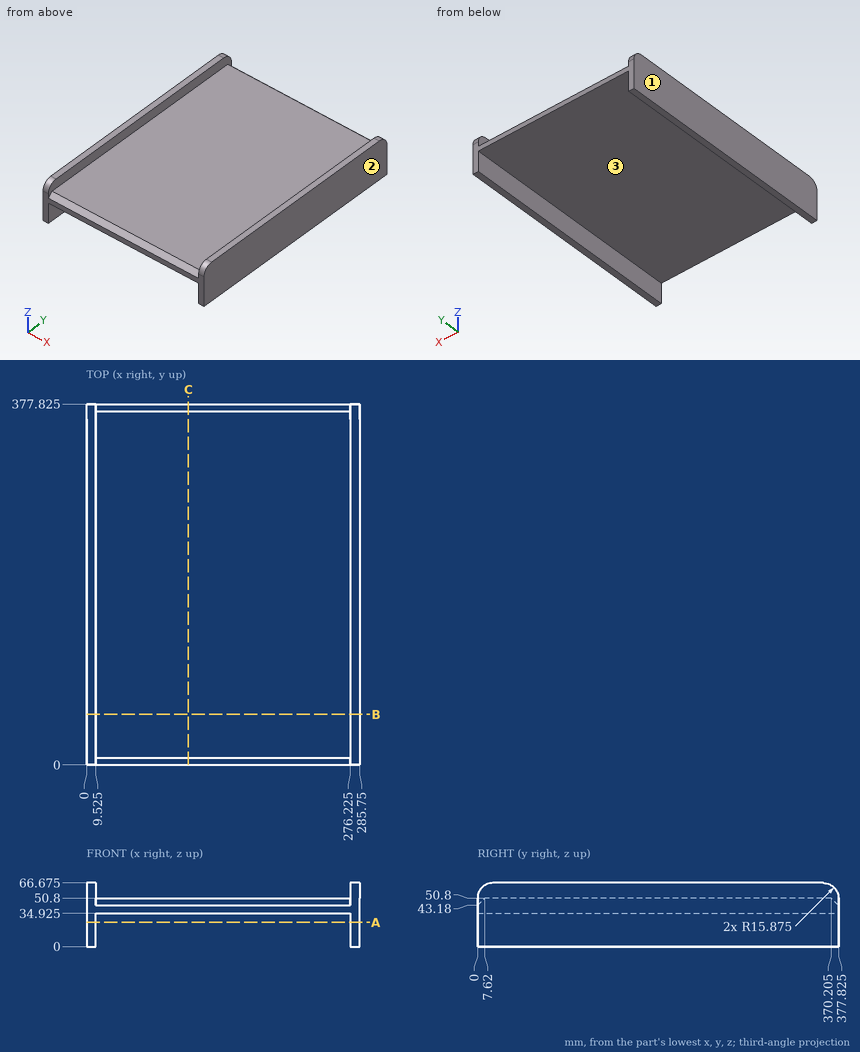
Geometry: see drawing. Coordinates: mm, zero at the bounding-box minimum. Give positions to 0.01 mm unless a question says otherwise; leave off trailing zeros. Write each loop counter-clockwise with the first axis right and the second up, starting at its lowest first coordinate (ties: lowest second). Pieces come first, ordered by that corner, then holes. Notation, with made-up numbers: M 62,-33 L 121,-33 A20 cw 121,-22 Z; hole C 53.5,58.25 d3. An arc over 180 degrees is marked long. Answer in a Markdown table with one row per item. Add a question column.
(1) Section C-C on x = 106.5. Return loops of the section in (y, z) (3 decimals), and give its area (3 significant figures).
(2) Section B-B on y = 53. Return loops of the section in (x, z) (3 decimals).
(3) First-contact query: pin 1 (1.5 mm diameter, centred on x = 189, y = 277, fed in from -Z) (3 decimals); pin 2 (2 mm diameter, centred on x = 70, y = 156, fed in from +Z); pin 3 (3 mm diameter, centred on y = 72.5, z = 32.5, fed in from -X). Flat tips, straight axial feed; report the tip coordinate or a pass-through.
(4) Section A-A on z = 25.5. Return loops of the section in (x, y) (3 decimals).
(5) Mould query, pull axis X, two halves, no side actions, for the marked faces 1, 2 and 3. Classes: +X half, -X half, draft (parallel to the pull), parting line (faces both ways), or undercut.
(6) Ray query, line 1 (X direction, y = 330, z = 22) (3 decimals); line 2 (Z direction, x = 189.5, y = 59) (3 decimals); line 3 (Y direction, x = 63, z = 49.5) (3 decimals). Return the intervals inside material, ascending.
Result set:
| question | item | result |
|---|---|---|
| 1 | outline | M 0,34.925 L 377.825,34.925 L 377.825,43.18 L 370.205,50.8 L 7.62,50.8 L 0,43.18 Z |
| 1 | area | 5,940 mm^2 |
| 2 | outline | M 0,0 L 9.525,0 L 9.525,34.925 L 276.225,34.925 L 276.225,0 L 285.75,0 L 285.75,66.675 L 276.225,66.675 L 276.225,50.8 L 9.525,50.8 L 9.525,66.675 L 0,66.675 Z |
| 3 | pin 1 | stops at z = 34.925 |
| 3 | pin 2 | stops at z = 50.8 |
| 3 | pin 3 | stops at x = 0 |
| 4 | outline | M 0,0 L 9.525,0 L 9.525,377.825 L 0,377.825 Z; M 276.225,0 L 285.75,0 L 285.75,377.825 L 276.225,377.825 Z |
| 5 | face 1 | -X half |
| 5 | face 2 | +X half |
| 5 | face 3 | undercut |
| 6 | line 1 | x = 0 to 9.525, 276.225 to 285.75 |
| 6 | line 2 | z = 34.925 to 50.8 |
| 6 | line 3 | y = 6.32 to 371.505 |
